Geometry check sheet. Reference: drawing and pictorial views, mm from the part's lowest x, y, z. Give positions to 0.01 mm unless a question says otherwise; leave off trailing zeros. Loops run counter-clockwise (first coordinate to the right, second up) from the corner with the lowest first, then second, coordinate; pieces in that order, holes last. Notation, with made-up numbers: (-31, 68.25) -> (-10, 68.25) arc R19 cw to (-10, 85.25) -> close; hole circle Ø5 at (-27.75, 66). An arc over 180 degrees is marked (long way). One line per item, written item: value. Start each with the question number.
(1) Scan lines: line 1 along Y through (x, z) = (111, 0.25) (1 decimal); line 2 along X through (y, z) = (94, 2.55); line 3 along Y through (x, z) = (133, 2) (1 decimal). Record each from-to range of solid material in increasing order. Write a range as from..to.
(2) Sectioned sample at A-A, the plane x = 70.5. Record the cut outline in (y, z).
(3) Gauge pin test, flat ends, axial feed: pin 1 Ø2.5 at (x, z) = (135, 3) entering from +Y; pin 2 Ø2.5 at (y, z) = (136, 2.5) entering from -X; pin 3 Ø2.5 at (y, z) = (3, 3.5) entering from +X (3 decimals). Record the tip position at first contact, or that the pin passes through.
(4) Sectioned sample at B-B, the plane z = 1.3. State how many separate pieces and enclosed holes the cut face has, then the cut area to 3 significant figures.
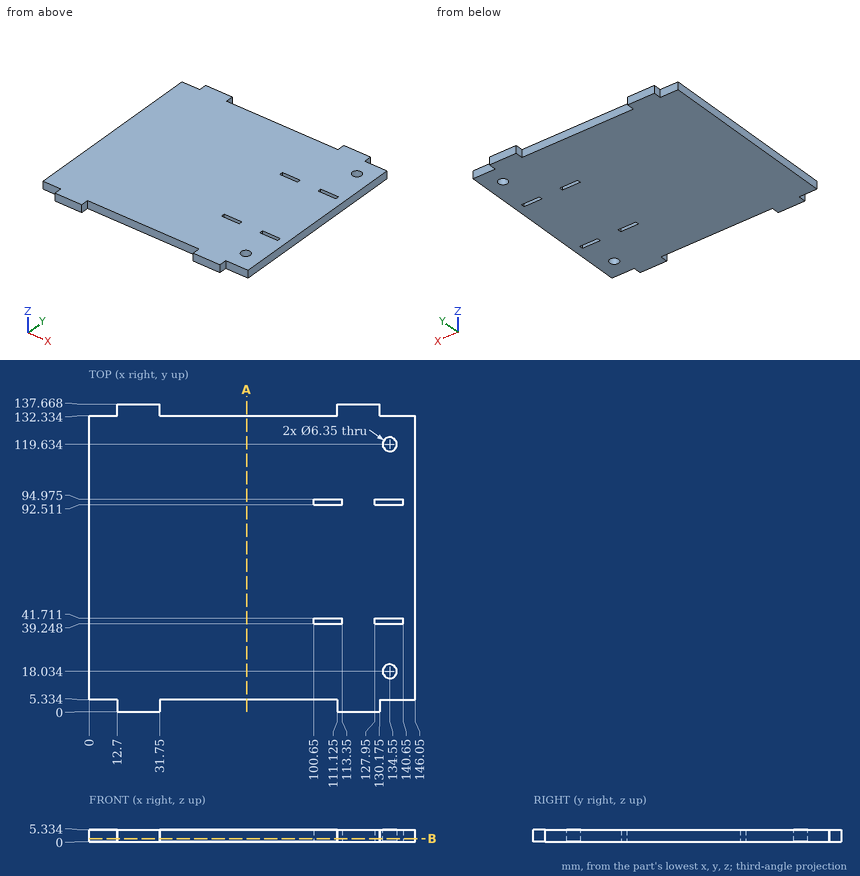
Calculated:
1. line 1: y = 5.3..39.2, 41.7..92.5, 95..132.3
1. line 2: x = 0..100.65, 113.35..127.95, 140.65..146.05
1. line 3: y = 5.3..15.3, 20.8..39.2, 41.7..92.5, 95..116.9, 122.4..132.3
2. outline: (5.33, 0) -> (132.33, 0) -> (132.33, 5.33) -> (5.33, 5.33) -> close
3. pin 1: stops at y = 132.33
3. pin 2: stops at x = 12.7
3. pin 3: stops at x = 130.175
4. separate pieces: 1
4. enclosed holes: 6
4. area: 18,800 mm2
